from build123d import *

# Parameters (mm, degrees)
F0_W      = 65
F0_H      = 30
F1_DEPTH  = 1.5
F2_R      = 1.5
F3_DEPTH  = 1.501
F4_R      = 3
F5_DEPTH  = 6
F6_R      = 0.2
F7_W      = 7.5
F7_H      = 13
F7_W_2    = 18
F7_W_3    = 10
F8_DEPTH  = 7
F9_W      = 15
F9_H      = 5
F10_DEPTH = 5


with BuildPart() as f1:
    # F0 (on Top) → F1 (new body)
    with BuildSketch(Plane.XY):
        Rectangle(F0_W, F0_H)
    extrude(amount=F1_DEPTH)

    # F2 (on face) → F3 (cut, through all)
    with BuildSketch(Plane.XY.offset(1.5)):
        with Locations((-29, 12)):
            Circle(F2_R)
        with Locations((-29, -12)):
            Circle(F2_R)
        with Locations((29, 12)):
            Circle(F2_R)
        with Locations((29, -12)):
            Circle(F2_R)
    extrude(amount=-F3_DEPTH, mode=Mode.SUBTRACT)

    # F4 (on face) → F5 (join)
    with BuildSketch(Plane.XY.offset(1.5)):
        with Locations((-27.5, 2)):
            Circle(F4_R)
        with Locations((-27.5, -5)):
            Circle(F4_R)
    extrude(amount=F5_DEPTH)

    # F6
    f6_edges = [f1.edges().sort_by_distance(p)[0] for p in [
        (-30.5, 2, 7.5),
        (-30.5, -5, 7.5),
    ]]
    fillet(f6_edges, radius=F6_R)

    # F7 (on face) → F8 (join)
    with BuildSketch(Plane.XY.offset(1.5)):
        with Locations((-20.75, 16.5)):
            Rectangle(F7_W, F7_H)
        with Locations((-10.25, 16.5)):
            Rectangle(F7_W, F7_H)
        with Locations((-15.5, -16.5)):
            Rectangle(F7_W_2, F7_H)
        with Locations((19.5, -16.5)):
            Rectangle(F7_W_3, F7_H)
        with Locations((8.5, -16.5)):
            Rectangle(F7_W_3, F7_H)
    extrude(amount=F8_DEPTH)

    # F9 (on face) → F10 (join)
    with BuildSketch(Plane.XY.offset(1.5)):
        with Locations((10, 10.5)):
            Rectangle(F9_W, F9_H)
    extrude(amount=F10_DEPTH)


solid = f1.part
Model file for the job. Use its own axes, mm. A direction names the side the tool comes from. Give positions to 0.01 mm unless a question says otherwise; leave off trailing zeros. Loops run counter-clockwise (first coordinate to the right, second up) from the corner with the lowest first, then second, coordinate; pieces in that order, holes last. Notation, with made-up numbers: (27, -8) -> (44, -8) arc R17 ccw to (44, 12) -> close; hole circle Ø2 at (-31, 67). An arc over 180 degrees is marked (long way). Use a Markdown table: item, result. Add a question column.
(1) Slice it at D-D on y = 2. List the corners of the cut face in (x, z).
(2) Mould opens along Y. For faces 1 (the flat face through (10, 13, 4)), 2 (the cylindrical face through (27.5, -11.93, 0.76)), 3 (the flat face through (19, -19, 1.5)) say: +Y half, -Y half, draft (parallel to the pull), parting line (faces both ways), or undercut.
(3) Slice it at A-A on y = -12. List the corners of the cut face in (x, z), and give its area (4 significant figures).
(4) Slice it at C-C on z = 5. List the corners of the cut face in (x, y), and give its area (3 significant figures).
(5) Drop flat-ended pins along their axis: pin 1 Ø4 at (x, y) = (6.5, -18) entering from -Z; pin 2 Ø1.5 at (x, z) = (11, 1.5) entering from +Y; pin 3 Ø3 at (y, z) = (-13, 4.5) entering from +X. Give the stop position or say it passes through.
(6) Slice it at B-B on x = 29. List the corners of the cut face in (y, z).
(7) Tool access for faces 4 (the flat face through (8, -10, 5)), 5 (the flat face through (24.5, -17, 5)), 6 (the flat face through (13.5, -17, 5)), 7 (the cylindrical face through (-30.5, -4.9, 4.4)): list every direction of +Z, -Z, +X, -X, +Y, -Y with a clear straight run to the whole face (end or side of a thin tool).
(8) Wall check: line 1 along Y through (x, z) = (-29, 0.4); line 2 along X through (y, z) = (-14, 4.5); line 3 along X through (y, z) = (16, 4.25). Give the ranges that are in metal, low to high.
Filled sheet:
| question | item | result |
|---|---|---|
| 1 | outline | (-32.5, 0) -> (32.5, 0) -> (32.5, 1.5) -> (-24.5, 1.5) -> (-24.5, 7.3) arc R0.2 ccw to (-24.7, 7.5) -> (-30.3, 7.5) arc R0.2 ccw to (-30.5, 7.3) -> (-30.5, 1.5) -> (-32.5, 1.5) -> close |
| 2 | face 1 | +Y half |
| 2 | face 2 | undercut |
| 2 | face 3 | draft |
| 3 | outline | (-32.5, 0) -> (-30.5, 0) -> (-30.5, 1.5) -> (-32.5, 1.5) -> close; (-27.5, 0) -> (27.5, 0) -> (27.5, 1.5) -> (24.5, 1.5) -> (24.5, 8.5) -> (14.5, 8.5) -> (14.5, 1.5) -> (13.5, 1.5) -> (13.5, 8.5) -> (3.5, 8.5) -> (3.5, 1.5) -> (-6.5, 1.5) -> (-6.5, 8.5) -> (-24.5, 8.5) -> (-24.5, 1.5) -> (-27.5, 1.5) -> close; (30.5, 0) -> (32.5, 0) -> (32.5, 1.5) -> (30.5, 1.5) -> close |
| 3 | area | 354.5 mm2 |
| 4 | outline | circle Ø6 at (-27.5, -5); circle Ø6 at (-27.5, 2); (-24.5, -23) -> (-6.5, -23) -> (-6.5, -10) -> (-24.5, -10) -> close; (-24.5, 10) -> (-17, 10) -> (-17, 23) -> (-24.5, 23) -> close; (-14, 10) -> (-6.5, 10) -> (-6.5, 23) -> (-14, 23) -> close; (2.5, 8) -> (17.5, 8) -> (17.5, 13) -> (2.5, 13) -> close; (3.5, -23) -> (13.5, -23) -> (13.5, -10) -> (3.5, -10) -> close; (14.5, -23) -> (24.5, -23) -> (24.5, -10) -> (14.5, -10) -> close |
| 4 | area | 821 mm2 |
| 5 | pin 1 | z = 1.5 |
| 5 | pin 2 | y = 15 |
| 5 | pin 3 | x = 24.5 |
| 6 | outline | (-15, 0) -> (-13.5, 0) -> (-13.5, 1.5) -> (-15, 1.5) -> close; (-10.5, 0) -> (10.5, 0) -> (10.5, 1.5) -> (-10.5, 1.5) -> close; (13.5, 0) -> (15, 0) -> (15, 1.5) -> (13.5, 1.5) -> close |
| 7 | face 4 | +Z, +X, -X |
| 7 | face 5 | +Z, +X, +Y, -Y |
| 7 | face 6 | +Z, -Y |
| 7 | face 7 | +Z |
| 8 | line 1 | -15 to -13.5, -10.5 to 10.5, 13.5 to 15 |
| 8 | line 2 | -24.5 to -6.5, 3.5 to 13.5, 14.5 to 24.5 |
| 8 | line 3 | -24.5 to -17, -14 to -6.5 |
